```python
from build123d import *

# Parameters (mm, degrees)
SKETCH2_R           = 5
BOSS_EXTRUDE1_DEPTH = 10
SKETCH3_R           = 10
SKETCH3_R_2         = 5
BOSS_EXTRUDE2_DEPTH = 76.2
BOSS_EXTRUDE3_START = 86.2
SKETCH2_2_R         = 5
BOSS_EXTRUDE3_DEPTH = 10
SKETCH5_R           = 65
BOSS_EXTRUDE4_DEPTH = 10
SKETCH6_R           = 55
CUT_EXTRUDE1_DEPTH  = 10
SKETCH7_R           = 80
CUT_EXTRUDE2_DEPTH  = 135.370532484
SKETCH8_R           = 10
BOSS_EXTRUDE6_DEPTH = 10


with BuildPart() as part:
    # Sketch2 → Boss-Extrude1 (new body)
    with BuildSketch(Plane.XY):
        with BuildLine():
            Line((-19.794866372, 2.857142857), (-9.897433186, 71.428571429))
            ThreePointArc((-9.897433186, 71.428571429), (0, 80), (9.897433186, 71.428571429))
            Line((9.897433186, 71.428571429), (19.794866372, 2.857142857))
            ThreePointArc((19.794866372, 2.857142857), (0, -20), (-19.794866372, 2.857142857))
        make_face()
        with Locations((0, 70)):
            Circle(SKETCH2_R, mode=Mode.SUBTRACT)
        with BuildLine():
            Line((-2.5, 9.682458366), (-2.5, 12))
            Line((-2.5, 12), (2.5, 12))
            Line((2.5, 12), (2.5, 9.682458366))
            ThreePointArc((2.5, 9.682458366), (0, -10), (-2.5, 9.682458366))
        make_face(mode=Mode.SUBTRACT)
    extrude(amount=BOSS_EXTRUDE1_DEPTH)

    # Sketch3 → Boss-Extrude2 (add)
    with BuildSketch(Plane.XY.offset(10)):
        with Locations(Location((0, 70, 0), (0, 0, 171.786789298))):
            Circle(SKETCH3_R)
        with Locations((0, 70)):
            Circle(SKETCH3_R_2, mode=Mode.SUBTRACT)
    extrude(amount=BOSS_EXTRUDE2_DEPTH)

    # Sketch2<2> → Boss-Extrude3 (add)
    with BuildSketch(Plane.XY.offset(BOSS_EXTRUDE3_START)):
        with BuildLine():
            Line((-19.794866372, 2.857142857), (-9.897433186, 71.428571429))
            ThreePointArc((-9.897433186, 71.428571429), (0, 80), (9.897433186, 71.428571429))
            Line((9.897433186, 71.428571429), (19.794866372, 2.857142857))
            ThreePointArc((19.794866372, 2.857142857), (0, -20), (-19.794866372, 2.857142857))
        make_face()
        with Locations((0, 70)):
            Circle(SKETCH2_2_R, mode=Mode.SUBTRACT)
        with BuildLine():
            Line((-2.5, 9.682458366), (-2.5, 12))
            Line((-2.5, 12), (2.5, 12))
            Line((2.5, 12), (2.5, 9.682458366))
            ThreePointArc((2.5, 9.682458366), (0, -10), (-2.5, 9.682458366))
        make_face(mode=Mode.SUBTRACT)
    extrude(amount=BOSS_EXTRUDE3_DEPTH)

    # Sketch5 → Boss-Extrude4 (add)
    with BuildSketch(Plane.XY.offset(96.2)):
        Circle(SKETCH5_R)
    extrude(amount=-BOSS_EXTRUDE4_DEPTH)

    # Sketch6 → Cut-Extrude1 (cut)
    with BuildSketch(Plane.XY.offset(96.2)):
        Circle(SKETCH6_R)
    extrude(amount=-CUT_EXTRUDE1_DEPTH, mode=Mode.SUBTRACT)

    # Sketch7 → Cut-Extrude2 (cut, through all)
    with BuildSketch(Plane(origin=(0, 0, 86.2), x_dir=(-1, 0, 0), z_dir=(0, 0, -1))):
        Circle(SKETCH7_R)
    extrude(amount=CUT_EXTRUDE2_DEPTH, mode=Mode.SUBTRACT)

    # Sketch8 → Boss-Extrude6 (add)
    with BuildSketch(Plane.XY.offset(96.2)):
        with BuildLine():
            Line((-19.69615506, 113.472963553), (-29.490777376, 57.924900084))
            ThreePointArc((-29.490777376, 57.924900084), (-20.457217444, 61.696857736), (-10.959640032, 64.06938653))
            Line((-10.959640032, 64.06938653), (-9.897433186, 71.428571429))
            ThreePointArc((-9.897433186, 71.428571429), (0, 80), (9.897433186, 71.428571429))
            Line((9.897433186, 71.428571429), (10.959640032, 64.06938653))
            ThreePointArc((10.959640032, 64.06938653), (20.457217444, 61.696857736), (29.490777376, 57.924900084))
            Line((29.490777376, 57.924900084), (19.69615506, 113.472963553))
            ThreePointArc((19.69615506, 113.472963553), (0, 130), (-19.69615506, 113.472963553))
        make_face()
        with Locations((0, 110)):
            Circle(SKETCH8_R, mode=Mode.SUBTRACT)
    extrude(amount=-BOSS_EXTRUDE6_DEPTH)


solid = part.part
```
Check sheet for the modelled part. Datum: model origin and axes. Units: mm. Give positions to 0.01 mm unless a question says otherwise; leave off trailing zeros. Write each loop counter-clockwise with the first axis right and the second up, starting at its lowest first coordinate (ties: lowest second). Pieces come first, ordered by that corner, then holes.
Item 1: Cross-section at B-B (x = 0). Enter the section's corners in (y, z).
Item 2: Draft check along Y on faces 1 (the face through (9, 55, 86.2)), 2 (the face through (-2.43, -64.955, 91.27)), 3 (the face through (-1.302, 119.915, 91.27)). Enter one of: released by +Y, released by -Y, zero draft, split by the parting line, or undercut.
Item 3: Gauge pin test, flat ends, axial feed: pin 1 (4 mm diameter, centred on y = 4.5, z = 88.5, fed in from -X); pin 2 (1 mm diameter, centred on x = -43.5, z = 93, fed in from -Y); pin 3 (3 mm diameter, centred on x = 30.5, z = 93, fed in from -Y). Record the tip position at first contact, or that the pin passes through.
Item 4: Cross-section at C-C (z = 94). Enter the section's corners in (x, y).
Item 5: Scan lines: L1, parallel to Y at x = -9, z = 92.75; L2, parallel to Y at x = 39, z = 90.25; L3, parallel to Y at x = -41, z = 92.5. Record each from-to range of solid material in increasing order.
Item 6: Cross-section at D-D (x = -46). Enter the section's corners in (y, z), and give its area (3 significant figures).
Item 7: Cross-section at A-A (y = 0). Enter the section's corners in (x, z).
Report:
1. outline: (-65, 86.2) - (-55, 86.2) - (-55, 96.2) - (-65, 96.2) - close; (55, 86.2) - (65, 86.2) - (65, 96.2) - (55, 96.2) - close; (75, 86.2) - (100, 86.2) - (100, 96.2) - (75, 96.2) - close; (120, 86.2) - (130, 86.2) - (130, 96.2) - (120, 96.2) - close
2. face 1: zero draft
2. face 2: split by the parting line
2. face 3: undercut
3. pin 1: stops at x = -64.95
3. pin 2: stops at y = -48.74
3. pin 3: stops at y = -58.17
4. outline: (-29.49, 57.92) arc R65 ccw (long way) to (29.49, 57.92) - (19.7, 113.47) arc R20 ccw to (-19.7, 113.47) - close; hole circle Ø110 at (0, 0); hole circle Ø20 at (0, 110); hole circle Ø10 at (0, 70)
5. L1: y = -64.37 to -54.26, 54.26 to 105.64, 114.36 to 127.86
5. L2: y = -52 to -38.78, 38.78 to 52
5. L3: y = -50.44 to -36.66, 36.66 to 50.44
6. outline: (-45.92, 86.2) - (-30.15, 86.2) - (-30.15, 96.2) - (-45.92, 96.2) - close; (30.15, 86.2) - (45.92, 86.2) - (45.92, 96.2) - (30.15, 96.2) - close
6. area: 315 mm2
7. outline: (-65, 86.2) - (-55, 86.2) - (-55, 96.2) - (-65, 96.2) - close; (55, 86.2) - (65, 86.2) - (65, 96.2) - (55, 96.2) - close
